from build123d import *

# Parameters (mm, degrees)
F1_DEPTH = 20
F2_R     = 4
F3_DEPTH = 7
F4_R     = 4
F5_DEPTH = 7


with BuildPart() as f1:
    # F0 (on Right) → F1 (new body)
    with BuildSketch(Plane.YZ):
        Polygon((0, 30), (0, 0), (30, 0), (30, 20), (50, 20), (50, 30), align=None)
    extrude(amount=F1_DEPTH)

    # F2 (on face) → F3 (join)
    with BuildSketch(Plane(origin=(0, 50, 0), x_dir=(-1, 0, 0), z_dir=(0, 1, 0))):
        with Locations((-10, 25)):
            Circle(F2_R)
    extrude(amount=F3_DEPTH)

    # F4 (on face) → F5 (join)
    with BuildSketch(Plane.XY.offset(30)):
        with Locations((10, 12.5)):
            Circle(F4_R)
    extrude(amount=F5_DEPTH)


solid = f1.part
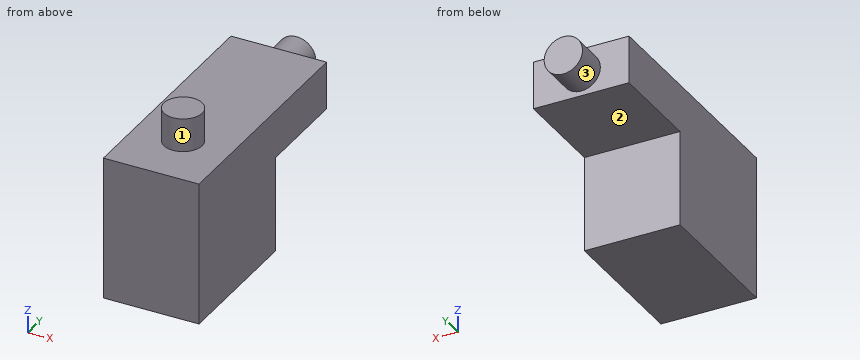
Design review of the part built by this model. Coordinates are the model's own, in mm. Face numbers are marked on the shaded views. A direction names the side the tool comes from. Round coordinates to 2 decimals unless told otherwise and drop trailing zeros. Write each loop counter-clockwise with the first axis right and the second up, starting at its lowest first coordinate (ties: lowest second). Pieces come first, ordered by that corner, then holes. Notation, with made-up numbers: (-34, -30) - (1, -30) arc R24 cw to (1, -18) - close; hole circle Ø2 at (59, 40.5). An arc over 180 degrees is marked (long way). Return JSON: item names as keys, results as strings. Group by question number.
Item 1: We need section A-A on z = 25. Write out the cut boundary in (x, y), and give its area (3 significant figures).
Item 2: We need section B-B on x = 10. Write out the cut boundary in (y, z).
Item 3: We need section D-D on z = 17.5. Write out the cut boundary in (x, y), and give its area (3 significant figures).
Item 4: For probe 1 along Y at (x, z) = (14.5, 21); probe 2 along Y at (x, z) = (2, 2); probe 3 along Z at (x, y) = (10.5, 30.5), list the stretches that pass through material, from the lowest coordinate up. Write a range as [from, to].
Item 5: We need section C-C on y = 12.5. Write out the cut boundary in (x, z), and give its area (3 significant figures).
Item 6: Machinability: for the marked faces 1, 2 and 3, which of the approach directions +Z, -Z, +X, -X, +Y, -Y give a long, thin tool a straight path to every point of the face, cutting with its end or side? Answer none if there is none.
Item 7: Insertion check: P1, Ø6, axis at x = 9.5, y = 36, coming from the +Z side; P2, Ø10, axis at x = 14, z = 14.5, coming from the +Y side; P3, Ø6, axis at x = 9, y = 44.5, coming from the -Z side. Each pin has a flat end and moves straight along its axis. Give the tip position at first contact, or say it passes through.
Model answer:
{
 "1": {"outline": "(0, 0) - (20, 0) - (20, 50) - (14, 50) - (14, 57) - (6, 57) - (6, 50) - (0, 50) - close", "area": "1,060 mm²"},
 "2": {"outline": "(0, 0) - (30, 0) - (30, 20) - (50, 20) - (50, 21) - (57, 21) - (57, 29) - (50, 29) - (50, 30) - (16.5, 30) - (16.5, 37) - (8.5, 37) - (8.5, 30) - (0, 30) - close"},
 "3": {"outline": "(0, 0) - (20, 0) - (20, 30) - (0, 30) - close", "area": "600 mm²"},
 "4": {"probe 1": "y = [0, 50]", "probe 2": "y = [0, 30]", "probe 3": "z = [20, 30]"},
 "5": {"outline": "(0, 0) - (20, 0) - (20, 30) - (14, 30) - (14, 37) - (6, 37) - (6, 30) - (0, 30) - close", "area": "656 mm²"},
 "6": {"face 1": "+Z", "face 2": "-Z, +X, -X, +Y", "face 3": "+Y"},
 "7": {"P1": "stops at z = 30", "P2": "stops at y = 30", "P3": "stops at z = 20"}
}
